```python
from build123d import *

# Parameters (mm, degrees)
F0_W      = 609.6
F0_H      = 254
F1_DEPTH  = 304.8
F2_W      = 101.6
F2_H      = 233.68
F3_DEPTH  = 5.08
F4_W      = 5.08
F4_H      = 254
F5_DEPTH  = 5.08
F6_W      = 91.44
F6_H      = 36.614052
F6_W_2    = 22.606
F6_H_2    = 20.32
F6_W_3    = 20.32
F7_DEPTH  = 5.08
F8_W      = 20.32
F8_H      = 222.552294
F9_DEPTH  = 12.7
F10_W     = 370.84
F10_H     = 177.8
F11_DEPTH = 5.08


with BuildPart() as f1:
    # F0 (on Front) → F1 (new body)
    with BuildSketch(Plane.XZ):
        with Locations((-17.430749, 23.316116)):
            Rectangle(F0_W, F0_H)
    extrude(amount=F1_DEPTH)

    # F2 (on face) → F3 (cut)
    with BuildSketch(Plane.XZ.offset(304.8)):
        with Locations((226.409251, 23.316116)):
            Rectangle(F2_W, F2_H)
    extrude(amount=-F3_DEPTH, mode=Mode.SUBTRACT)

    # F4 (on face) → F5 (cut)
    with BuildSketch(Plane.XZ.offset(304.8)):
        with Locations((162.909251, 23.316116)):
            Rectangle(F4_W, F4_H)
    extrude(amount=-F5_DEPTH, mode=Mode.SUBTRACT)

    # F6 (on face) → F7 (join)
    with BuildSketch(Plane.XZ.offset(299.72)):
        with Locations((226.409251, 116.76909)):
            Rectangle(F6_W, F6_H)
        with Locations((199.612251, 75.602064)):
            Rectangle(F6_W_2, F6_H_2)
        with Locations((227.679251, 75.602064)):
            Rectangle(F6_W_3, F6_H_2)
        with Locations((254.349251, 75.602064)):
            Rectangle(F6_W_3, F6_H_2)
        with Locations((198.469251, 42.582064)):
            Rectangle(F6_W_3, F6_H_2)
        with Locations((227.679251, 42.582064)):
            Rectangle(F6_W_3, F6_H_2)
        with Locations((254.349251, 42.582064)):
            Rectangle(F6_W_3, F6_H_2)
        with Locations((198.469251, 9.562064)):
            Rectangle(F6_W_3, F6_H_2)
        with Locations((225.393251, 9.562064)):
            Rectangle(F6_W_3, F6_H_2)
        with Locations((254.349251, 9.562064)):
            Rectangle(F6_W_3, F6_H_2)
        with Locations((225.139251, -23.457936)):
            Rectangle(F6_W_3, F6_H_2)
    extrude(amount=F7_DEPTH)

    # F8 (on face) → F9 (join)
    with BuildSketch(Plane.XZ.offset(304.8)):
        with Locations((134.969251, 22.832263)):
            Rectangle(F8_W, F8_H)
    extrude(amount=F9_DEPTH)

    # F10 (on face) → F11 (cut)
    with BuildSketch(Plane.XZ.offset(304.8)):
        with Locations((-98.710749, 23.316116)):
            Rectangle(F10_W, F10_H)
    extrude(amount=-F11_DEPTH, mode=Mode.SUBTRACT)


solid = f1.part
```
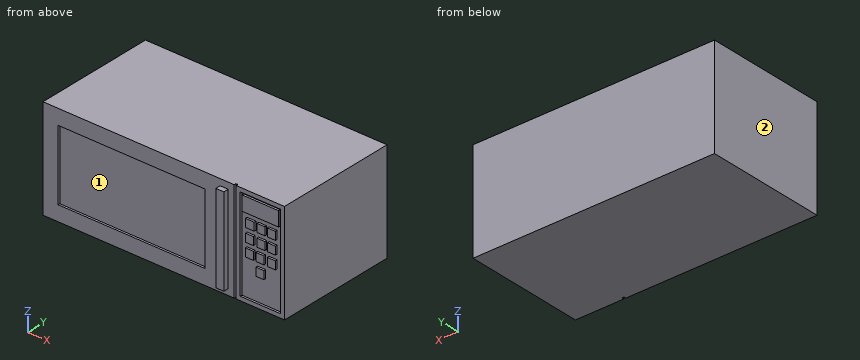
Geometry check sheet. Reference: the model listing, model coordinates, mm. Face numbers are marked on the shaded views. A direction names the side the tool comes from. Coordinates: 2 decimals unless noted, no trailing zeros. Order: outer loops, then holes, each group sorted by start corner. A loop starts at its lowest first (then second) coordinate and runs counter-clockwise, first axis right, second up. Notation, with made-up numbers: (-13.5, -2.75) - (0.5, -2.75) arc R19 ccw to (0.5, 1.25) - close; hole circle Ø6 at (-11, -29). An arc over 180 degrees is marked (long way). Use one line per item in the form item = value.
1. Section check B-B (x = -80). Record the boundary of the cut face in (y, z).
Here are the results:
outline = (-304.8, -103.68) - (0, -103.68) - (0, 150.32) - (-304.8, 150.32) - (-304.8, 112.22) - (-299.72, 112.22) - (-299.72, -65.58) - (-304.8, -65.58) - close
2. Gauge pin test, flat ends, axial feed: pin 1 (4 mm diameter, centred on x = 27.5, z = -13.5, fed in from +Y); pin 2 (18.5 mm diameter, centred on x = 210, z = 121.5, fed in from -Y); pin 3 (6.5 mm diameter, centred on x = 131, y = -312.5, fed in from +Z); pin 4 (10 mm diameter, centred on x = -256, z = -4.5, fed in from -Y). Record the tip position at first contact, or that the pin passes through.
Here are the results:
pin_1 = 0
pin_2 = -304.8
pin_3 = 134.11
pin_4 = -299.72
3. Section check A-A (z = -72). Record the boundary of the cut face in (x, y), then the cut area to 3 significant figures.
Here are the results:
outline = (-322.23, -304.8) - (124.81, -304.8) - (124.81, -317.5) - (145.13, -317.5) - (145.13, -304.8) - (160.37, -304.8) - (160.37, -299.72) - (165.45, -299.72) - (165.45, -304.8) - (175.61, -304.8) - (175.61, -299.72) - (277.21, -299.72) - (277.21, -304.8) - (287.37, -304.8) - (287.37, 0) - (-322.23, 0) - close
area = 186,000 mm²
4. Scan lines: line 1 (Y direction, x = -206, z = 107); line 2 (Z direction, x = -227, y = -303); line 3 (Y direction, x = 109, z = 81.5). Record each from-to range of solid material in increasing order.
Here are the results:
line_1 = -299.72 to 0
line_2 = -103.68 to -65.58, 112.22 to 150.32
line_3 = -304.8 to 0
5. Access from +Z, -Z, +X, -X, +Y, -Y to the whole of each face (thin tool, end or side, straight path). Record for the marked faces 1 and 2.
Here are the results:
face_1 = -Y
face_2 = +Z, -Z, -X, +Y, -Y
